Geometry: final body of the model. Coordinates: model frame, mm. A direction names the side the tool comes from. Give positions to 0.01 mm unless a question says otherwise; leave off trailing zeros. Order: outer loops, then holes, each group sorted by start corner. A loop starts at its lowest first (then second) coordinate and runs counter-clockwise, first axis right, second up. Notation, with made-up numbers: (81.25, 86.25) -> (124.25, 86.25) arc R20 cw to (124.25, 118.25) -> close; hole circle Ø4 at (50.25, 87.25). An arc over 180 degrees is marked (long way). Answer in a Markdown table with one row per item. Add a question column.
Q1. Contact query for flat-ended pins moving along their axis: P1, Ø8, axis at y = 34.5, z = -1, coming from the +X side; P2, Ø5, axis at x = -1, y = 23.5, coming from the +Z side. Output: stop coordinate, or through.
Q2. Line query: line 1 along Y through (x, z) = (-4.5, 2.5); line 2 along Y through (x, z) = (-1.25, -7); line 3 along Y through (x, z) = (6.75, -0.5). Output: solid intervals per line, ascending. Write a range as from..to.
Q3. Cut plane B-B on z = 0. Return the cut outline in (x, y), and give its area (3 significant figures).
Q4. Cut plane C-C on y = 28. Return the cut outline in (x, z), and give its area (3 significant figures).
Q5. Set-up query: faces 5 (the face through (6.466, 3.042, -2.681)), 6 (the face through (6.466, 19.647, -2.681)), 7 (the face through (3, 30, -3)), 8 (the face through (0, 0, 0)). Return all of +Z, -Z, +X, -X, +Y, -Y with unobstructed straight access to the full face (end or side cutting, diameter ignored); none if empty.
Q6. Pull-direction query (Y, two-part tool) for faces 1 (the face through (0, 43, 0)), 2 (the face through (0, 6, -7.3)), 3 (the face through (6.466, 38.056, -2.681)), 4 (the face through (-3, 34, -3)); classes: +Y half, -Y half, draft (parallel to the pull), parting line (faces both ways), or undercut.
Q7. Cut plane A-A on x = 0. Return the cut outline in (y, z).
from build123d import *

# Parameters (mm, degrees)
CHAMFER1_SIZE = 1


with BuildPart() as part:
    # Sketch1 → Revolve1 (revolve)
    with BuildSketch(Plane.XY):
        Polygon((0, 0), (7, 0), (7, 6), (9, 6), (9, 9), (7, 9), (7, 30), (3.75, 30), (3.75, 34), (7, 34), (7, 43), (0, 43), align=None)
    revolve(axis=Axis((0, 43, 0), (0, -1, 0)))

    # Chamfer1
    chamfer1_edges = [part.edges().sort_by_distance(p)[0] for p in [
        (-7, 43, 0),
    ]]
    chamfer(chamfer1_edges, length=CHAMFER1_SIZE)


solid = part.part
Completed:
| question | item | result |
|---|---|---|
| 1 | P1 | stops at x = 7 |
| 1 | P2 | stops at z = 7 |
| 2 | line 1 | y = 0..30, 34..43 |
| 2 | line 2 | y = 6..9 |
| 2 | line 3 | y = 0..30, 34..42.23 |
| 3 | outline | (-9, 6) -> (-7, 6) -> (-7, 0) -> (7, 0) -> (7, 6) -> (9, 6) -> (9, 9) -> (7, 9) -> (7, 30) -> (3.75, 30) -> (3.75, 34) -> (7, 34) -> (7, 42) -> (6, 43) -> (-6, 43) -> (-7, 42) -> (-7, 34) -> (-3.75, 34) -> (-3.75, 30) -> (-7, 30) -> (-7, 9) -> (-9, 9) -> close |
| 3 | area | 587 mm² |
| 4 | outline | circle Ø14 at (0, 0) |
| 4 | area | 154 mm² |
| 5 | face 5 | -Y |
| 5 | face 6 | +Y |
| 5 | face 7 | none |
| 5 | face 8 | +Z, -Z, +X, -X, -Y |
| 6 | face 1 | +Y half |
| 6 | face 2 | -Y half |
| 6 | face 3 | draft |
| 6 | face 4 | undercut |
| 7 | outline | (0, -7) -> (6, -7) -> (6, -9) -> (9, -9) -> (9, -7) -> (30, -7) -> (30, -3.75) -> (34, -3.75) -> (34, -7) -> (42, -7) -> (43, -6) -> (43, 6) -> (42, 7) -> (34, 7) -> (34, 3.75) -> (30, 3.75) -> (30, 7) -> (9, 7) -> (9, 9) -> (6, 9) -> (6, 7) -> (0, 7) -> close |
